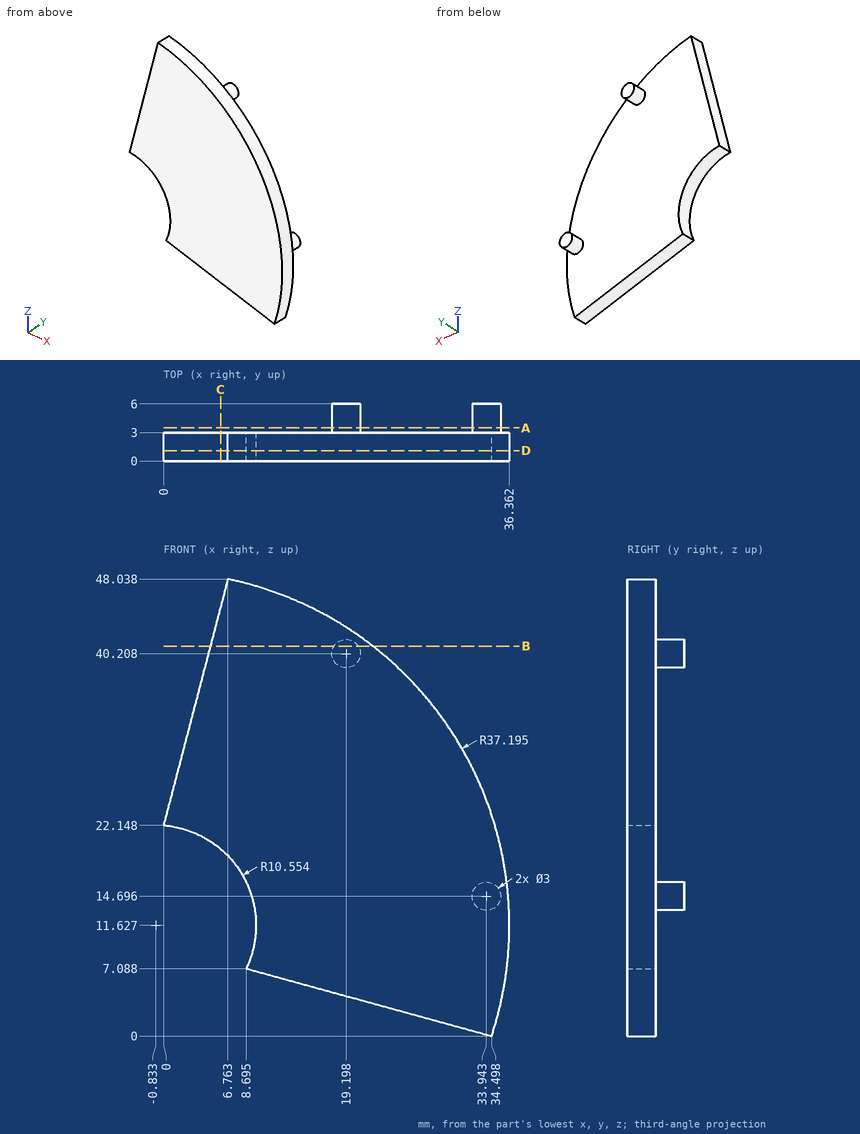
Answer from the drawing. Dimensions are ordinates in mm from the lowest x, y and z of the part. Give positions to 0.01 mm unless a question says otherwise; leave off trailing zeros. Order: outer loops, then holes, each group sorted by start corner. A loop starts at its lowest first (then second) coordinate and runs counter-clockwise, first axis right, second up. Notation, with made-up numbers: (79.25, 26) -> (136.25, 26) arc R20 ccw to (136.25, 55) -> close; hole circle Ø1 at (62.5, 57.25). An arc over 180 degrees is marked (long way). Answer as a JSON object with one key per item and string values. Group by question number.
1. Consider line 1 along Y through (x, z) = (11, 28.5); line 2 along X through (y, z) = (1.5, 42.5) (1 decimal); line 3 along Z through (x, y) = (15, 2.65) (1 decimal). Determine where each line is inside the solid, lowest interval first. Write a range as [from, to].
2. Section D-D on y = 1.1 is taken. Determine the outline of the cut face in (x, z) (1 decimal).
3. Section A-A on y = 3.5 is taken. Determine the outline of the cut face in (x, z) (1 decimal).
4. Section B-B on z = 41 is taken. Determine the outline of the cut face in (x, y) (1 decimal).
5. Section C-C on x = 6 is taken. Determine the outline of the cut face in (y, z).
6. Flat-ended cylindrical pins translate along their axes: pin 1 Ø18 at (x, z) = (9.5, 18.5) entering from +Y; pin 2 Ø1.5 at (y, z) = (1.5, 9.5) entering from -X; pin 3 Ø1.5 at (y, z) = (2.5, 32.5) entering from -X. Find the tip coordinate at first contact, or state that the pin passes through.
Result sheet:
{
 "1": {"line 1": "y = [0, 3]", "line 2": "x = [5.3, 19.9]", "line 3": "z = [5.4, 45.3]"},
 "2": {"outline": "(0, 22.1) arc R10.6 cw to (8.7, 7.1) -> (34.5, 0) arc R37.2 ccw to (6.8, 48) -> close"},
 "3": {"outline": "circle Ø3 at (19.2, 40.2); circle Ø3 at (33.9, 14.7)"},
 "4": {"outline": "(4.9, 0) -> (22, 0) -> (22, 3) -> (20.5, 3) -> (20.5, 6) -> (17.9, 6) -> (17.9, 3) -> (4.9, 3) -> close"},
 "5": {"outline": "(0, 19.67) -> (3, 19.67) -> (3, 45.12) -> (0, 45.12) -> close"},
 "6": {"pin 1": "stops at y = 3", "pin 2": "stops at x = 9.32", "pin 3": "stops at x = 2.51"}
}
